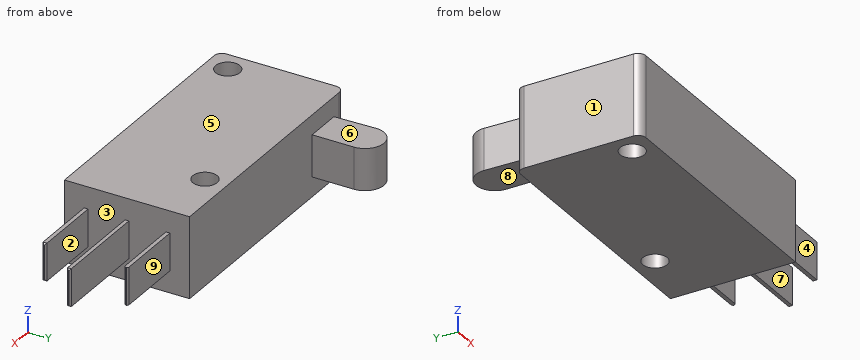
```python
from build123d import *

# Parameters (mm, degrees)
F0_R     = 1.55
F1_DEPTH = 10.3
F3_DEPTH = 2.5
F4_DEPTH = 2.5
F5_W     = 0.5
F5_H     = 4.75
F6_DEPTH = 9
F5_W_2   = 0.474308
F7_DEPTH = 12.5
F8_SIZE  = 0.2
F9_R     = 1


with BuildPart() as f1:
    # F0 (on Top) → F1 (new body)
    with BuildSketch(Plane.XY):
        Polygon((-23.728283, -19.735446), (-25.866954, -19.735446), (-25.866954, -35.635446), (7.133046, -35.635446), (7.133046, -19.735446), (-19.066954, -19.735446), align=None)
        with Locations((-23.066954, -32.835446)):
            Circle(F0_R, mode=Mode.SUBTRACT)
        with Locations((-0.866954, -22.535446)):
            Circle(F0_R, mode=Mode.SUBTRACT)
        with BuildLine():
            Line((-23.866123, -14.498595), (-23.728283, -19.735446))
            Line((-23.728283, -19.735446), (-19.066954, -19.735446))
            Line((-19.066954, -19.735446), (-19.066954, -14.435446))
            ThreePointArc((-19.066954, -14.435446), (-21.435376, -16.835239), (-23.866123, -14.498595))
        make_face()
        with BuildLine():
            ThreePointArc((-19.066954, -14.435446), (-21.498531, -12.035654), (-23.866123, -14.498595))
            ThreePointArc((-23.866123, -14.498595), (-21.435376, -16.835239), (-19.066954, -14.435446))
        make_face()
    extrude(amount=F1_DEPTH)

    # F2 (on face) → F3 (cut)
    with BuildSketch(Plane.XY.offset(10.3)):
        with BuildLine():
            Line((-23.866123, -14.498595), (-23.728283, -19.735446))
            Line((-23.728283, -19.735446), (-19.066954, -19.735446))
            Line((-19.066954, -19.735446), (-19.066954, -14.435446))
            ThreePointArc((-19.066954, -14.435446), (-21.498531, -12.035654), (-23.866123, -14.498595))
        make_face()
    extrude(amount=-F3_DEPTH, mode=Mode.SUBTRACT)

    # F0 (on Top) → F4 (cut)
    with BuildSketch(Plane.XY):
        with BuildLine():
            Line((-23.866123, -14.498595), (-23.728283, -19.735446))
            Line((-23.728283, -19.735446), (-19.066954, -19.735446))
            Line((-19.066954, -19.735446), (-19.066954, -14.435446))
            ThreePointArc((-19.066954, -14.435446), (-21.435376, -16.835239), (-23.866123, -14.498595))
        make_face()
        with BuildLine():
            ThreePointArc((-19.066954, -14.435446), (-21.498531, -12.035654), (-23.866123, -14.498595))
            ThreePointArc((-23.866123, -14.498595), (-21.435376, -16.835239), (-19.066954, -14.435446))
        make_face()
    extrude(amount=F4_DEPTH, mode=Mode.SUBTRACT)

    # F5 (on face) → F6 (join)
    with BuildSketch(Plane.YZ.offset(7.133046)):
        with Locations((-22.485446, 5.15)):
            Rectangle(F5_W, F5_H)
        with Locations((-32.885446, 5.15)):
            Rectangle(F5_W, F5_H)
    extrude(amount=F6_DEPTH)

    # F5 (on face) → F7 (join)
    with BuildSketch(Plane.YZ.offset(7.133046)):
        with Locations((-27.698292, 5.15)):
            Rectangle(F5_W_2, F5_H)
    extrude(amount=F7_DEPTH)

    # F8
    f8_edges = [f1.edges().sort_by_distance(p)[0] for p in [
        (16.133046, -22.235446, 5.15),
        (16.133046, -22.735446, 5.15),
        (19.633046, -27.461138, 5.15),
        (19.633046, -27.698292, 7.525),
        (19.633046, -27.935446, 5.15),
        (19.633046, -27.698292, 2.775),
        (16.133046, -32.635446, 5.15),
        (16.133046, -32.885446, 7.525),
        (16.133046, -33.135446, 5.15),
        (16.133046, -32.885446, 2.775),
    ]]
    chamfer(f8_edges, length=F8_SIZE)

    # F9
    f9_edges = [f1.edges().sort_by_distance(p)[0] for p in [
        (-25.866954, -19.735446, 5.15),
        (-25.866954, -35.635446, 5.15),
    ]]
    fillet(f9_edges, radius=F9_R)


solid = f1.part
```
Design review of the part built by this model. Coordinates are the model's own, in mm. Face numbers are marked on the shaded views. A direction names the side the tool comes from. Give positions to 0.01 mm unless a question says otherwise; leave off trailing zeros. Write each loop counter-clockwise with the first axis right and the second up, starting at its lowest first coordinate (ties: lowest second). Pieces come first, ordered by that corner, then holes.
(1) Tool access review of the marked faces 5, 6, 7, 8 and 9: name each direction out of +Z, -Z, +X, -X, +Y, -Y from which nothing blocks a thin tool from reaching the whole face with its end or side.
Checked values:
face 5: +Z, +X, -X, +Y, -Y
face 6: +Z, +X, -X, +Y
face 7: +Z, -Z, +X
face 8: -Z, +X, -X, +Y
face 9: +Z, -Z, +X, +Y
(2) Clearance check with flat-ended pins moving along their axes: pin 1 Ø2.5 at (x, z) = (11.5, 4.5) entering from -Y; pin 2 Ø4 at (x, y) = (-20.5, -16) entering from -Z; pin 3 Ø0.6 at (x, y) = (12.5, -33) entering from -Z (3 decimals). State where each tip first meets the part, or that it passes through.
Checked values:
pin 1: stops at y = -33.14
pin 2: stops at z = 2.5
pin 3: stops at z = 2.775
(3) Mouldability with a two-part tool opening along Y and no side actions: class the marked faces 1, 2, 3 and 4 as +Y half, -Y half, draft (parallel to the pull), parting line (faces both ways), or undercut.
Checked values:
face 1: draft
face 2: undercut
face 3: undercut
face 4: -Y half
(4) Add section A-A (x = 14). Give the boundary of the cut face in (y, z) (3 decimals), and give its area (3 significant figures).
Checked values:
outline: (-33.135, 2.775) - (-32.635, 2.775) - (-32.635, 7.525) - (-33.135, 7.525) - close; (-27.935, 2.775) - (-27.461, 2.775) - (-27.461, 7.525) - (-27.935, 7.525) - close; (-22.735, 2.775) - (-22.235, 2.775) - (-22.235, 7.525) - (-22.735, 7.525) - close
area: 7.00 mm2
(5) Add section C-C (y = -32). Give the boundary of the cut face in (x, z).
Checked values:
outline: (-25.87, 0) - (-24.37, 0) - (-24.37, 10.3) - (-25.87, 10.3) - close; (-21.76, 0) - (7.13, 0) - (7.13, 10.3) - (-21.76, 10.3) - close
(6) Wall thickness on line 1 along Y through (x, z) = (15, 6.75); line 2 along Y through (x, z) = (-19, 8.5); line 3 along Z through (x, y) = (-19.5, -17.25): over which ranges is each line inside the solid? List them lowest first.
Checked values:
line 1: y = -33.14 to -32.64, -27.94 to -27.46, -22.74 to -22.24
line 2: y = -35.64 to -19.74
line 3: z = 2.5 to 7.8
(7) Add section B-B (z = 5.75). Give the number of separate pieces and of enclosed holes in the cut face, and give its area (3 significant figures).
Checked values:
separate pieces: 1
enclosed holes: 2
area: 558 mm2
(8) Add section D-D (z = 8.5). Give the boundary of the cut face in (x, y), and give its area (3 significant figures).
Checked values:
outline: (-25.87, -34.64) arc R1 ccw to (-24.87, -35.64) - (7.13, -35.64) - (7.13, -19.74) - (-24.87, -19.74) arc R1 ccw to (-25.87, -20.74) - close; hole circle Ø3.1 at (-23.07, -32.84); hole circle Ø3.1 at (-0.87, -22.54)
area: 509 mm2
